Verification items for this drawing (mm, ordinates from the low corner). Coordinates: 2 decimals unless noted, no trailing zeros. Order: outer loops, then holes, each group sorted by start corner. A loop starts at its lowest first (then second) coordinate and runs counter-clockwise, first axis right, second up. Notation, with made-up numbers: M -18,17 L 7,17 A32 cw 7,51 Z; hole C 50.5,25 d11. An arc over 180 degrees is marked long. Write item = value, one per line.
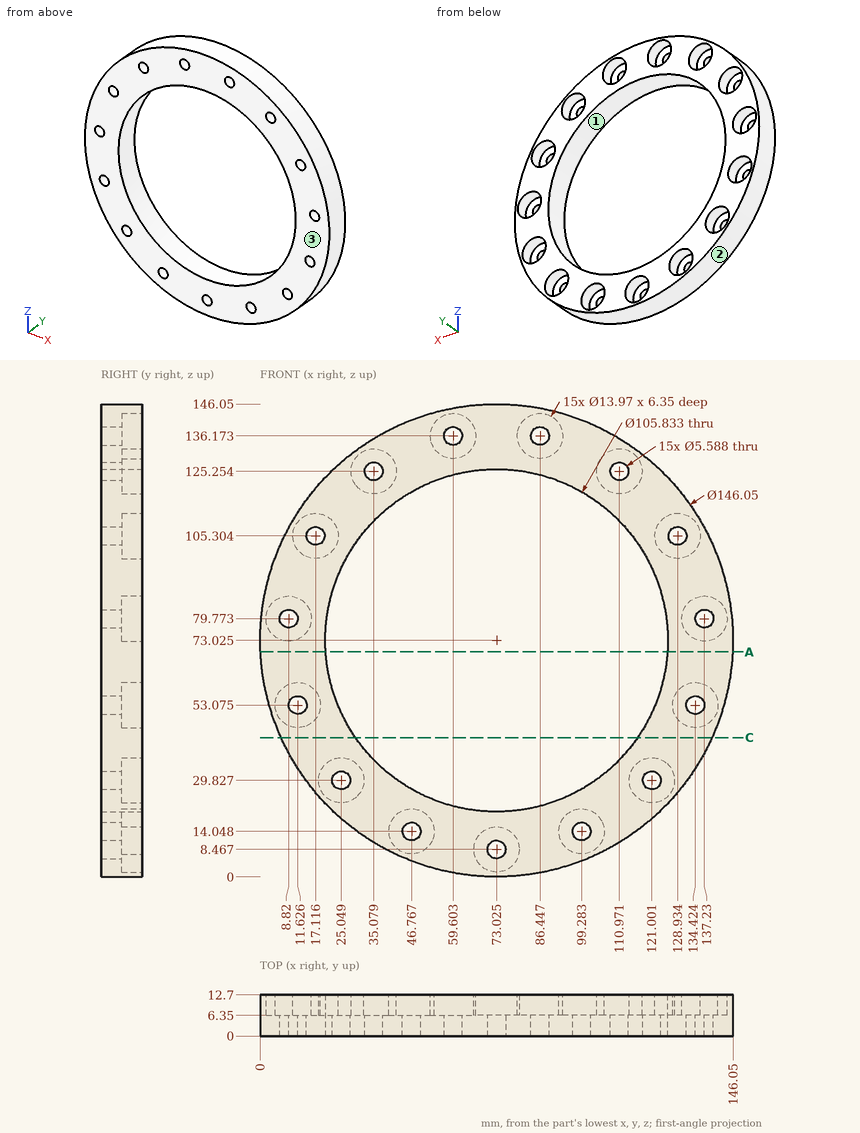
Item 1: Sectioned sample at C-C, the plane z = 43. Enter the section's corners in (x, y), then the cut area to 3 significant figures.
Report:
outline = M 6.46,0 L 29.45,0 L 29.45,12.7 L 6.46,12.7 Z; M 116.6,0 L 139.59,0 L 139.59,12.7 L 116.6,12.7 Z
area = 584 mm^2
Item 2: Sectioned sample at A-A, the plane z = 69.5. Enter the section's corners in (x, y) (1 decimal).
Report:
outline = M 0.1,0 L 20.2,0 L 20.2,12.7 L 0.1,12.7 Z; M 125.8,0 L 146,0 L 146,12.7 L 125.8,12.7 Z
Item 3: Gauge pin test, flat ends, axial feed: pin 1 (3 mm diameter, centred on x = 48, y = 6.5, fed in from -Z); pin 2 (6 mm diameter, centred on x = 17.5, y = 8, fed in from +Z); pin 3 (5 mm diameter, centred on y = 10, z = 25, fed in from +X). Record the tip position at first contact, or that the pin passes through.
Report:
pin_1 = 3.89
pin_2 = 123.76
pin_3 = 130.12
Item 4: Release check for a two-part mould opening along Z. For the marked faces 1, 2 and 3 record: pulls with the +Z half, pulls with the -Z half, needs draft (parallel to the pull), parting line crosses it, or undercut.
Report:
face_1 = undercut
face_2 = parting line crosses it
face_3 = needs draft
Item 5: Scan lines: L1, parallel to Z at x = 132, y = 12 (1 decimal); L2, parallel to Z at x = 64, y = 10.5 (1 decimal); L3, parallel to Z at x = 48.5, y = 5 (1 decimal). Record each from-to range of solid material in increasing order. Write a range as from..to.
Report:
L1 = 30..46.5, 59.6..75.1, 84.4..99, 111.6..116.1
L2 = 0.6..20.9, 125.2..130.7, 141.6..145.5
L3 = 4.2..11.9, 16.2..26.1, 119.9..141.8
